from build123d import *

# Parameters (mm, degrees)
BOSS_EXTRUDE1_DEPTH = 25
SKETCH2_W           = 1
SKETCH2_H           = 74
SKETCH2_W_2         = 31.5
SKETCH2_H_2         = 1
CUT_EXTRUDE1_DEPTH  = 23
CHAMFER1_SIZE       = 0.5


with BuildPart() as part:
    # Sketch1 → Boss-Extrude1 (new body)
    with BuildSketch(Plane(origin=(0, 0, 0), x_dir=(1, 0, 0), z_dir=(0, 1, 0))):
        Polygon((-18.647540984, 3.790983607), (-18.647540984, -21.209016393), (12.852459016, -21.209016393), (12.852459016, 78.790983607), (-11.647540984, 78.790983607), (-11.647540984, 3.790983607), align=None)
    extrude(amount=BOSS_EXTRUDE1_DEPTH)

    # Sketch2 → Cut-Extrude1 (cut)
    with BuildSketch(Plane(origin=(0, 25, 0), x_dir=(1, 0, 0), z_dir=(0, 1, 0))):
        with Locations((-9.147540984, 41.790983607)):
            Rectangle(SKETCH2_W, SKETCH2_H)
        with Locations((-6.347540984, 41.790983607)):
            Rectangle(SKETCH2_W, SKETCH2_H)
        with Locations((-3.547540984, 41.790983607)):
            Rectangle(SKETCH2_W, SKETCH2_H)
        with Locations((-0.747540984, 41.790983607)):
            Rectangle(SKETCH2_W, SKETCH2_H)
        with Locations((2.052459016, 41.790983607)):
            Rectangle(SKETCH2_W, SKETCH2_H)
        with Locations((4.852459016, 41.790983607)):
            Rectangle(SKETCH2_W, SKETCH2_H)
        with Locations((7.652459016, 41.790983607)):
            Rectangle(SKETCH2_W, SKETCH2_H)
        with Locations((10.452459016, 41.790983607)):
            Rectangle(SKETCH2_W, SKETCH2_H)
        Polygon((-11.647540984, 4.790983607), (-11.647540984, 3.790983607), (12.852459016, 3.790983607), (12.852459016, 4.790983607), (10.952459016, 4.790983607), (9.952459016, 4.790983607), (8.152459016, 4.790983607), (7.152459016, 4.790983607), (5.352459016, 4.790983607), (4.352459016, 4.790983607), (2.552459016, 4.790983607), (1.552459016, 4.790983607), (-0.247540984, 4.790983607), (-1.247540984, 4.790983607), (-3.047540984, 4.790983607), (-4.047540984, 4.790983607), (-5.847540984, 4.790983607), (-6.847540984, 4.790983607), (-8.647540984, 4.790983607), (-9.647540984, 4.790983607), align=None)
        with Locations((-2.897540984, 1.290983607)):
            Rectangle(SKETCH2_W_2, SKETCH2_H_2)
        with Locations((-2.897540984, -1.509016393)):
            Rectangle(SKETCH2_W_2, SKETCH2_H_2)
        with Locations((-2.897540984, -4.309016393)):
            Rectangle(SKETCH2_W_2, SKETCH2_H_2)
        with Locations((-2.897540984, -7.109016393)):
            Rectangle(SKETCH2_W_2, SKETCH2_H_2)
        with Locations((-2.897540984, -9.909016393)):
            Rectangle(SKETCH2_W_2, SKETCH2_H_2)
        with Locations((-2.897540984, -18.309016393)):
            Rectangle(SKETCH2_W_2, SKETCH2_H_2)
        with Locations((-2.897540984, -15.509016393)):
            Rectangle(SKETCH2_W_2, SKETCH2_H_2)
        with Locations((-2.897540984, -12.709016393)):
            Rectangle(SKETCH2_W_2, SKETCH2_H_2)
    extrude(amount=-CUT_EXTRUDE1_DEPTH, mode=Mode.SUBTRACT)

    # Chamfer1
    chamfer1_edges = [part.edges().sort_by_distance(p)[0] for p in [
        (5.352459016, 25, -41.790983607),
        (6.252459016, 25, -4.790983607),
        (8.152459016, 25, -41.790983607),
        (9.052459016, 25, -4.790983607),
        (10.952459016, 25, -41.790983607),
        (11.902459016, 25, -4.790983607),
        (-10.647540984, 25, -4.790983607),
        (-9.647540984, 25, -41.790983607),
        (9.952459016, 25, -41.790983607),
        (7.152459016, 25, -41.790983607),
        (4.352459016, 25, -41.790983607),
        (1.552459016, 25, -41.790983607),
        (-1.247540984, 25, -41.790983607),
        (-4.047540984, 25, -41.790983607),
        (-2.897540984, 25, 21.209016393),
        (-6.847540984, 25, -41.790983607),
        (-2.897540984, 25, -1.790983607),
        (-2.897540984, 25, -0.790983607),
        (12.852459016, 25, 20.009016393),
        (-2.897540984, 25, 1.009016393),
        (-2.897540984, 25, 2.009016393),
        (-2.897540984, 25, 3.809016393),
        (-2.897540984, 25, 4.809016393),
        (-2.897540984, 25, 6.609016393),
        (-2.897540984, 25, 7.609016393),
        (-2.897540984, 25, 12.209016393),
        (-2.897540984, 25, 13.209016393),
        (-18.647540984, 25, 0.109016393),
        (-2.897540984, 25, 15.009016393),
        (-2.897540984, 25, 16.009016393),
        (-18.647540984, 25, 2.909016393),
        (-2.897540984, 25, 17.809016393),
        (-2.897540984, 25, 18.809016393),
        (-18.647540984, 25, 5.709016393),
        (-2.897540984, 25, 9.409016393),
        (11.902459016, 25, -78.790983607),
        (-2.897540984, 25, 10.409016393),
        (-18.647540984, 25, 8.509016393),
        (-18.647540984, 25, 11.309016393),
        (-18.647540984, 25, 14.109016393),
        (-18.647540984, 25, 16.909016393),
        (-18.647540984, 25, 20.009016393),
        (12.852459016, 25, 16.909016393),
        (12.852459016, 25, 14.109016393),
        (-11.647540984, 25, -41.790983607),
        (12.852459016, 25, 11.309016393),
        (12.852459016, 25, 8.509016393),
        (12.852459016, 25, 5.709016393),
        (12.852459016, 25, 2.909016393),
        (12.852459016, 25, 0.109016393),
        (12.852459016, 25, -2.790983607),
        (12.852459016, 25, -41.790983607),
        (9.052459016, 25, -78.790983607),
        (6.252459016, 25, -78.790983607),
        (3.452459016, 25, -78.790983607),
        (0.652459016, 25, -78.790983607),
        (-2.147540984, 25, -78.790983607),
        (-4.947540984, 25, -78.790983607),
        (-7.747540984, 25, -78.790983607),
        (-10.647540984, 25, -78.790983607),
        (-2.897540984, 25, -3.790983607),
        (-8.647540984, 25, -41.790983607),
        (-7.747540984, 25, -4.790983607),
        (-18.647540984, 25, -2.790983607),
        (-5.847540984, 25, -41.790983607),
        (-4.947540984, 25, -4.790983607),
        (-3.047540984, 25, -41.790983607),
        (-2.147540984, 25, -4.790983607),
        (-0.247540984, 25, -41.790983607),
        (0.652459016, 25, -4.790983607),
        (2.552459016, 25, -41.790983607),
        (3.452459016, 25, -4.790983607),
    ]]
    chamfer(chamfer1_edges, length=CHAMFER1_SIZE)


solid = part.part
Geometry: final body of the model. Coordinates: model frame, mm. A direction names the side the tool comes from. Give positions to 0.01 mm unless a question says otherwise; leave off trailing zeros. Answer in a Markdown table with one row per item.
(1) Set-up query: faces 4 (the flat face through (-8, 13, -4.791)), 5 (the flat face through (-8.648, 13, -41)), 6 (the flat face through (-11.648, 12, -42)). Return all of +Z, -Z, +X, -X, +Y, -Y with unobstructed straight access to the full face (end or side cutting, diameter ignored); none if empty.
Answers below:
| item | result |
|---|---|
| face 4 | +X, -X, +Y |
| face 5 | -Z, +Y |
| face 6 | -Z, -X, +Y, -Y |
(2) Draft query along Z for faces 1 (the flat face through (-4.048, 13, -41)), 2 (the flat face through (1, 12, -78.791)), 3 (the flat face through (-3, 13, 16.009)). Return one class per face: +Z half, -Z half, draft (parallel to the pull), parting line (faces both ways), or undercut.
Answers below:
| item | result |
|---|---|
| face 1 | draft |
| face 2 | -Z half |
| face 3 | undercut |
(3) Section query A-A on y = 12.25. State how many separate pieces and enclosed holes the cut face has, then the cut area to 3 significant figures.
Answers below:
| item | result |
|---|---|
| separate pieces | 18 |
| enclosed holes | 0 |
| area | 1,760 mm^2 |
(4) Pin query (flat end, axial travel): pin 1 (5 mm diameter, centred on y = 7.5, z = -45.5, fed in from -X); pin 2 (1.1 mm diameter, centred on x = -6.5, z = 13, fed in from +Y). Return the tip coordinate at first contact, or that it passes through.
Answers below:
| item | result |
|---|---|
| pin 1 | x = -11.65 |
| pin 2 | y = 24.84 |
(5) Ray query, line 1 along Y through (x, z) = (5, -50); line 2 along Y through (x, z) = (0, -33). Return the intervals inside material, ascending. Write a range as [from, to].
Answers below:
| item | result |
|---|---|
| line 1 | [0, 2] |
| line 2 | [0, 24.75] |
